from build123d import *

# Parameters (mm, degrees)
SKETCH1_W           = 60
SKETCH1_H           = 78
BOSS_EXTRUDE1_DEPTH = 3
SKETCH2_W           = 8
SKETCH2_H           = 78
BOSS_EXTRUDE2_DEPTH = 25
SKETCH5_R           = 2
CUT_EXTRUDE2_DEPTH  = 30
SKETCH6_R           = 12.5
CUT_EXTRUDE3_DEPTH  = 29


with BuildPart() as part:
    # Sketch1 → Boss-Extrude1 (new body)
    with BuildSketch(Plane(origin=(0, 0, 0), x_dir=(1, 0, 0), z_dir=(0, 1, 0))):
        Rectangle(SKETCH1_W, SKETCH1_H)
    extrude(amount=BOSS_EXTRUDE1_DEPTH)

    # Sketch2 → Boss-Extrude2 (add)
    with BuildSketch(Plane(origin=(0, 3, 0), x_dir=(1, 0, 0), z_dir=(0, 1, 0))):
        with Locations((26, 0)):
            Rectangle(SKETCH2_W, SKETCH2_H)
    extrude(amount=BOSS_EXTRUDE2_DEPTH)

    # Sketch5 → Cut-Extrude2 (cut)
    with BuildSketch(Plane.ZY.offset(-22)):
        with Locations((35, 10)):
            Circle(SKETCH5_R)
        with Locations((-35, 10)):
            Circle(SKETCH5_R)
    extrude(amount=-CUT_EXTRUDE2_DEPTH, mode=Mode.SUBTRACT)

    # Sketch6 → Cut-Extrude3 (cut, through all)
    with BuildSketch(Plane(origin=(0, 0, 0), x_dir=(-1, 0, 0), z_dir=(0, -1, 0))):
        with Locations((2, 0)):
            Circle(SKETCH6_R)
    extrude(amount=-CUT_EXTRUDE3_DEPTH, mode=Mode.SUBTRACT)


solid = part.part
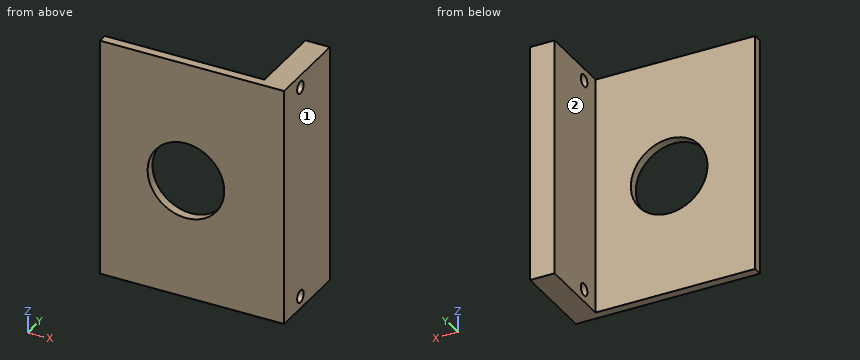
Could you check a few things on this model? Use its own coordinates, in mm. Face numbers are marked on the shaded views. A direction names the side the tool comes from. Give positions to 0.01 mm unless a question says otherwise; leave off trailing zeros. Order: outer loops, then holes, each group sorted by start corner. A loop starts at its lowest first (then second) coordinate and runs counter-clockwise, first axis right, second up.
1. Which directions (+Z, -Z, +X, -X, +Y, -Y) give clear straight access to the entire face, cutting with the end or side of a thin tool? Please do the marked faces 1 and 2.
Answers below:
face 1: +Z, -Z, +X, +Y, -Y
face 2: +Z, -Z, -X, +Y
2. Suppose I cut it at D-D (z = 7.5). Write out the boundary of the cut face in (x, y).
Answers below:
outline: (-30, 0) - (-12, 0) - (-12, 3) - (-30, 3) - close; (8, 0) - (30, 0) - (30, 28) - (22, 28) - (22, 3) - (8, 3) - close
3. I need wall thicknesses on L1, parallel to X at y = 1.65, z = 0; L2, parallel to Y at x = 25.25, z = -35; L3, parallel to Z at x = -2, y = 1.65. Which ranges of each line are inside material? Lowest first, please.
Answers below:
L1: x = -30 to -14.5, 10.5 to 30
L2: y = 0 to 8, 12 to 28
L3: z = -39 to -12.5, 12.5 to 39
4. Suppose I cut it at C-C (x = -2). Write out the boundary of the cut face in (y, z), plus the area to 3 significant figures.
Answers below:
outline: (0, -39) - (3, -39) - (3, -12.5) - (0, -12.5) - close; (0, 12.5) - (3, 12.5) - (3, 39) - (0, 39) - close
area: 159 mm2
5. Suppose I cut it at A-A (z = 35). Write out the boundary of the cut face in (x, y).
Answers below:
outline: (-30, 0) - (30, 0) - (30, 8) - (22, 8) - (22, 3) - (-30, 3) - close; (22, 12) - (30, 12) - (30, 28) - (22, 28) - close
6. Suppose I cut it at B-B (y = 10). Write out the boundary of the cut face in (x, z).
Answers below:
outline: (22, -39) - (30, -39) - (30, -37) - (22, -37) - close; (22, -33) - (30, -33) - (30, 33) - (22, 33) - close; (22, 37) - (30, 37) - (30, 39) - (22, 39) - close
7. For pin 1 (6.5 mm diameter, centred on y = 10, z = 35, fed in from -X); pin 2 (2 mm diameter, centred on x = 20, z = -8, fed in from +Y), each with a flat end and sliding along its axis, tell me the tip position at first contact or that it passes through.
Answers below:
pin 1: stops at x = 22
pin 2: stops at y = 3
